The model under review builds one solid part; all positions refer to its coordinate system, in mm. Face numbers are marked on the shaded views. A direction names the side the tool comes from. Round coordinates to 2 decimals unless told otherwise and drop trailing zeros. Loops run counter-clockwise (first coordinate to the right, second up) from the corner with the lowest first, then second, coordinate; pieces in that order, holes last. Notation, with made-up numbers: (22.25, -31.75) -> (35.25, -31.75) arc R32 ccw to (35.25, -5.75) -> close; hole circle Ø7 at (51.25, -0.5). An arc over 180 degrees is marked (long way). Return JSON: item names as keys, results as strings. Group by question number.
```python
from build123d import *

# Parameters (mm, degrees)
CYLINDER002_R     = 1.5
CYLINDER002_DEPTH = 10
CYLINDER001_R     = 1.5
CYLINDER001_DEPTH = 10
PAD002_DEPTH      = 5
PAD001_DEPTH      = 20
SKETCH008_R       = 2.1
POCKET002_DEPTH   = 7
SKETCH009_R       = 3.6
POCKET003_DEPTH   = 2
CYLINDER_R        = 8
CYLINDER_DEPTH    = 5
SKETCH_R          = 10
SKETCH_R_2        = 6.7
PAD_DEPTH         = 25
FILLET_R          = 5
FILLET001_R       = 3
CHAMFER_SIZE      = 1
CHAMFER001_SIZE   = 1


with BuildPart() as zylinder002:
    # Cylinder002 → Cylinder002 (new body)
    with BuildSketch(Plane(origin=(6.5, -7, 0), x_dir=(1, 0, 0), z_dir=(0, 0, 1))):
        Circle(CYLINDER002_R)
    extrude(amount=CYLINDER002_DEPTH)


with BuildPart() as zylinder001:
    # Cylinder001 → Cylinder001 (new body)
    with BuildSketch(Plane(origin=(-6.5, -7, 15), x_dir=(1, 0, 0), z_dir=(0, 0, 1))):
        Circle(CYLINDER001_R)
    extrude(amount=CYLINDER001_DEPTH)


with BuildPart() as pad002:
    # Sketch011 → Pad002 (new body)
    with BuildSketch(Plane.XY.offset(20)):
        with BuildLine():
            Line((-10, 0), (-10, -15))
            Line((10, -15), (-10, -15))
            Line((10, 0), (10, -15))
            ThreePointArc((-10, 0), (0, -10), (10, 0))
        make_face()
    extrude(amount=PAD002_DEPTH)


with BuildPart() as pocket003:
    # Sketch003 → Pad001 (new body)
    with BuildSketch(Plane.XY):
        with BuildLine():
            ThreePointArc((-10, 0), (0, -10), (10, 0))
            Line((10, 0), (10, -8))
            Line((10, -8), (25, -8))
            Line((25, -8), (25, -15))
            Line((-25, -15), (25, -15))
            Line((-25, -8), (-25, -15))
            Line((-10, -8), (-25, -8))
            Line((-10, 0), (-10, -8))
        make_face()
    extrude(amount=PAD001_DEPTH)

    # Sketch008 → Pocket002 (cut)
    with BuildSketch(Plane.XZ.offset(15)):
        with Locations((-17.5, 10)):
            Circle(SKETCH008_R)
        with Locations((17.5, 10)):
            Circle(SKETCH008_R)
    extrude(amount=-POCKET002_DEPTH, mode=Mode.SUBTRACT)

    # Sketch009 → Pocket003 (cut)
    with BuildSketch(Plane(origin=(0, -8, 0), x_dir=(-1, 0, 0), z_dir=(0, 1, 0))):
        with Locations((-17.5, 10)):
            Circle(SKETCH009_R)
        with Locations((17.5, 10)):
            Circle(SKETCH009_R)
    extrude(amount=-POCKET003_DEPTH, mode=Mode.SUBTRACT)


with BuildPart() as zylinder:
    # Cylinder → Cylinder (new body)
    with BuildSketch(Plane.XY.offset(10)):
        Circle(CYLINDER_R)
    extrude(amount=CYLINDER_DEPTH)


with BuildPart() as chamfer001:
    # Sketch → Pad (new body)
    with BuildSketch(Plane.XY):
        Circle(SKETCH_R)
        Circle(SKETCH_R_2, mode=Mode.SUBTRACT)
    extrude(amount=PAD_DEPTH)

    # Cut: cut Zylinder
    add(zylinder.part, mode=Mode.SUBTRACT)

    # Fusion: union Pad002, Pocket003
    add(pad002.part)
    add(pocket003.part)

    # Cut001: cut Zylinder001
    add(zylinder001.part, mode=Mode.SUBTRACT)

    # Cut002: cut Zylinder002
    add(zylinder002.part, mode=Mode.SUBTRACT)

    # Fillet
    fillet_edges = [chamfer001.edges().sort_by_distance(p)[0] for p in [
        (25, -11.5, 20),
        (-25, -11.5, 20),
    ]]
    fillet(fillet_edges, radius=FILLET_R)

    # Fillet001
    fillet001_edges = [chamfer001.edges().sort_by_distance(p)[0] for p in [
        (10, -15, 22.5),
        (-10, -15, 22.5),
    ]]
    fillet(fillet001_edges, radius=FILLET001_R)

    # Chamfer
    chamfer_edges = [chamfer001.edges().sort_by_distance(p)[0] for p in [
        (-6.7, 0, 10),
    ]]
    chamfer(chamfer_edges, length=CHAMFER_SIZE)

    # Chamfer001
    chamfer001_edges = [chamfer001.edges().sort_by_distance(p)[0] for p in [
        (-6.7, 0, 15),
    ]]
    chamfer(chamfer001_edges, length=CHAMFER001_SIZE)


solid = chamfer001.part
```
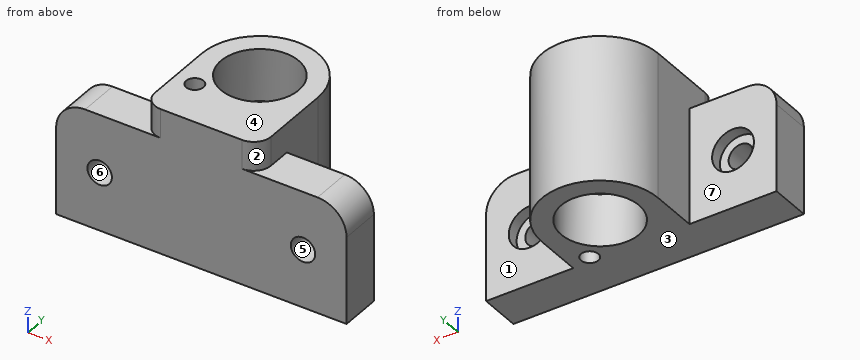
1. Draft analysis for pull direction Z (two halves, no side actions). For the marked faces 4, 5, 6 and 7, state which applies: pulls with the +Z half, pulls with the -Z half, needs draft (parallel to the pull), parting line crosses it, or undercut.
2. Wall thickness on line 1 (Z direction, x = -17.5, y = -12.2); line 2 (Z direction, x = 7, y = -3.5); line 3 (X direction, y = 0, z = 18.75): over which ranges is each line inside the solid? List them lowest first.
3. We need section C-C, the plane x = 17.5. Write out the cut boundary in (y, z), then the cut area to 3 significant figures.
4. We need section A-A, the plane x = 0. Write out the cut boundary in (y, z).
5. For P1, Ø4, axis at x = 17.5, z = 10, coming from the -Y side (3 decimals); P2, Ø3, axis at y = -5.5, z = 11, coming from the -X side; P3, Ø1.5, axis at x = 12, z = 17, coming from the +Y side; P4, Ø6, axis at x = -10.5, z = 21, coming from the +Y side, all flat-tipped, find the tip position at first contact; note any pin that passes through.
6. Tool access review of the marked faces 1, 2 and 3: name each direction out of +Z, -Z, +X, -X, +Y, -Y from which nothing blocks a thin tool from reaching the whole face with its end or side.
7. We need section D-D, the plane x = 11. Write out the cut boundary in (y, z), then the cut area to 3 significant figures.
8. We need section B-B, the plane z = 22. Write out the cut boundary in (x, y).
Check sheet entries:
{
 "1": {"face 4": "pulls with the +Z half", "face 5": "undercut", "face 6": "undercut", "face 7": "needs draft"},
 "2": {"line 1": "z = 0 to 7.9, 12.1 to 20", "line 2": "z = 0 to 10, 15 to 25", "line 3": "x = -10 to -6.7, 6.7 to 10"},
 "3": {"outline": "(-15, 0) -> (-8, 0) -> (-8, 6.4) -> (-10, 6.4) -> (-10, 7.9) -> (-15, 7.9) -> close; (-15, 12.1) -> (-10, 12.1) -> (-10, 13.6) -> (-8, 13.6) -> (-8, 20) -> (-15, 20) -> close", "area": "105 mm²"},
 "4": {"outline": "(-15, 0) -> (-6.7, 0) -> (-6.7, 9) -> (-7.7, 10) -> (-8, 10) -> (-8, 15) -> (-7.7, 15) -> (-6.7, 16) -> (-6.7, 25) -> (-15, 25) -> close; (6.7, 0) -> (10, 0) -> (10, 25) -> (6.7, 25) -> (6.7, 16) -> (7.7, 15) -> (8, 15) -> (8, 10) -> (7.7, 10) -> (6.7, 9) -> close"},
 "5": {"P1": "passes through", "P2": "stops at x = -10", "P3": "stops at y = -8", "P4": "stops at y = 6.61"},
 "6": {"face 1": "+Z, -Z, +X, +Y", "face 2": "+Z, +X, -Y", "face 3": "-Z, +X, -X, +Y, -Y"},
 "7": {"outline": "(-15, 0) -> (-8, 0) -> (-8, 20) -> (-15, 20) -> close", "area": "140 mm²"},
 "8": {"outline": "(-10, -12) arc R3 ccw to (-7, -15) -> (7, -15) arc R3 ccw to (10, -12) -> (10, 0) arc R10 ccw to (-10, 0) -> close; hole circle Ø3 at (-6.5, -7); hole circle Ø13.4 at (0, 0)"}
}
